Check sheet for the modelled part. Datum: model origin and axes. Units: mm. Face numbers are marked on the shaded views. A direction names the side the tool comes from. Round coordinates to 2 decimals unless told otherwise and drop trailing zeros. Order: outer loops, then holes, each group sorted by start corner. A loop starts at its lowest first (then second) coordinate and runs counter-clockwise, first axis right, second up. Notation, with made-up numbers: (-17.75, -11) -> (-4.75, -11) arc R27 cw to (-4.75, 18) -> close; hole circle Ø4 at (49, 19.5). An arc over 180 degrees is marked (long way). Answer in a Markdown table with one row per item.
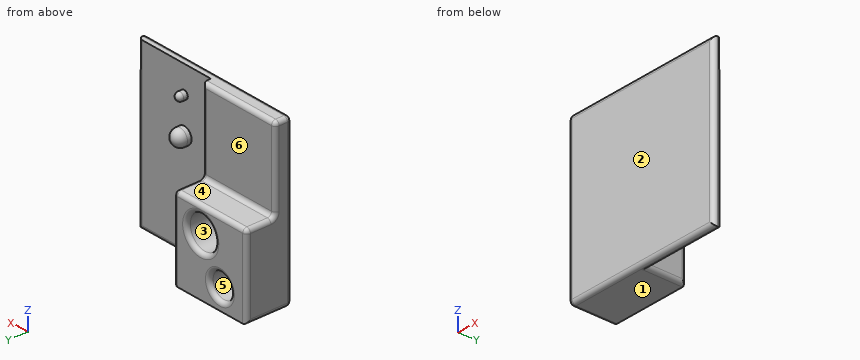
from build123d import *

# Parameters (mm, degrees)
SKETCH1_W           = 10
SKETCH1_H           = 20
BOSS_EXTRUDE1_DEPTH = 2
SKETCH2_W           = 10
SKETCH2_H           = 20
BOSS_EXTRUDE2_DEPTH = 1
SKETCH3_R           = 0.5
BOSS_EXTRUDE3_DEPTH = 1
FILLET1_R           = 0.5
SKETCH4_R           = 1
BOSS_EXTRUDE4_DEPTH = 1.5
FILLET2_R           = 1
SKETCH5_W           = 10
SKETCH5_H           = 10
BOSS_EXTRUDE5_DEPTH = 3.5
SKETCH7_R           = 1.5
CUT_EXTRUDE1_DEPTH  = 4
SKETCH8_R           = 2
CUT_EXTRUDE2_DEPTH  = 5
FILLET3_R           = 0.5


with BuildPart() as part:
    # Sketch1 → Boss-Extrude1 (new body)
    with BuildSketch(Plane(origin=(0, 0, 0), x_dir=(1, 0, 0), z_dir=(0, 1, 0))):
        with Locations((5, 10)):
            Rectangle(SKETCH1_W, SKETCH1_H)
    extrude(amount=BOSS_EXTRUDE1_DEPTH)

    # Sketch2 → Boss-Extrude2 (add)
    with BuildSketch(Plane(origin=(0, 0, 0), x_dir=(1, 0, 0), z_dir=(0, 1, 0))):
        with Locations((15, 10)):
            Rectangle(SKETCH2_W, SKETCH2_H)
    extrude(amount=BOSS_EXTRUDE2_DEPTH)

    # Sketch3 → Boss-Extrude3 (add)
    with BuildSketch(Plane(origin=(0, 1, 0), x_dir=(1, 0, 0), z_dir=(0, 1, 0))):
        with Locations(Location((13.691502903, 3.252748725, 0), (0, 0, 90))):
            Circle(SKETCH3_R)
    extrude(amount=BOSS_EXTRUDE3_DEPTH)

    # Fillet1
    fillet1_edges = [part.edges().sort_by_distance(p)[0] for p in [
        (13.691502903, 2, -2.752748725),
    ]]
    fillet(fillet1_edges, radius=FILLET1_R)

    # Sketch4 → Boss-Extrude4 (add)
    with BuildSketch(Plane(origin=(0, 1, 0), x_dir=(1, 0, 0), z_dir=(0, 1, 0))):
        with Locations(Location((13.672959069, 7.53387034, 0), (0, 0, 90))):
            Circle(SKETCH4_R)
    extrude(amount=BOSS_EXTRUDE4_DEPTH)

    # Fillet2
    fillet2_edges = [part.edges().sort_by_distance(p)[0] for p in [
        (13.672959069, 2.5, -6.53387034),
    ]]
    fillet(fillet2_edges, radius=FILLET2_R)

    # Sketch5 → Boss-Extrude5 (add)
    with BuildSketch(Plane(origin=(0, 2, 0), x_dir=(1, 0, 0), z_dir=(0, 1, 0))):
        with Locations((5, 15)):
            Rectangle(SKETCH5_W, SKETCH5_H)
    extrude(amount=BOSS_EXTRUDE5_DEPTH)

    # Sketch7 → Cut-Extrude1 (cut)
    with BuildSketch(Plane(origin=(0, 5.5, 0), x_dir=(1, 0, 0), z_dir=(0, 1, 0))):
        with Locations(Location((3.651027896, 17.503330669, 0), (0, 0, 270))):
            Circle(SKETCH7_R)
    extrude(amount=-CUT_EXTRUDE1_DEPTH, mode=Mode.SUBTRACT)

    # Sketch8 → Cut-Extrude2 (cut)
    with BuildSketch(Plane(origin=(0, 5.5, 0), x_dir=(1, 0, 0), z_dir=(0, 1, 0))):
        with Locations(Location((6.300805509, 13.043308943, 0), (0, 0, 270))):
            Circle(SKETCH8_R)
    extrude(amount=-CUT_EXTRUDE2_DEPTH, mode=Mode.SUBTRACT)

    # Fillet3
    fillet3_edges = [part.edges().sort_by_distance(p)[0] for p in [
        (0, 2, -5),
        (20, 0, -10),
        (20, 1, -10),
        (10, 0, -20),
        (0, 0, -10),
        (10, 0, 0),
        (0, 1, 0),
        (5, 2, 0),
        (5, 2, -10),
        (10, 2, -5),
        (15, 1, -20),
        (0, 2.75, -20),
        (10, 3.25, -20),
        (10, 5.5, -15),
        (10, 3.75, -10),
        (0, 3.75, -10),
        (0, 5.5, -15),
        (5, 5.5, -10),
        (6.300805509, 5.5, -15.043308943),
        (3.651027896, 5.5, -19.003330669),
    ]]
    fillet(fillet3_edges, radius=FILLET3_R - 0.0001)  # a hair under: the kernel refuses the full size


solid = part.part
Item 1: Cross-section at B-B (y = 4.3). Record the boundary of the cut face in (x, z), and give its area (3 significant figures).
Result sheet:
| item | result |
|---|---|
| outline | (0, -19.5) arc R0.5 ccw to (0.5, -20) -> (9.5, -20) arc R0.5 ccw to (10, -19.5) -> (10, -10.5) arc R0.5 ccw to (9.5, -10) -> (0.5, -10) arc R0.5 ccw to (0, -10.5) -> close; hole circle Ø3 at (3.65, -17.5); hole circle Ø4 at (6.3, -13.04) |
| area | 80.2 mm^2 |
Item 2: Depth check by flat-ended pin: P1, Ø5, axis at x = 6.3, z = -13.04, coming from the +Y side; P2, Ø7.5, axis at x = 14, z = -11, coming from the +Y side; P3, Ø1.5, axis at x = 16.5, z = -2, coming from the +Y side; P4, Ø4, axis at x = 6, z = -5.5, coming from the +Y side. Enter the tip coordinate at first touch or a pass-through.
Result sheet:
| item | result |
|---|---|
| P1 | stops at y = 5.5 |
| P2 | stops at y = 2.5 |
| P3 | stops at y = 1 |
| P4 | stops at y = 2 |
Item 3: Set-up check for the marked faces 4, 5 and 6: record each of +Z, -Z, +X, -X, +Y, -Y from which the full face is reachable in a straight line by a thin tool's end or side.
Result sheet:
| item | result |
|---|---|
| face 4 | +Z, +X, -X, +Y |
| face 5 | +Y |
| face 6 | +Z, -X, +Y |
Item 4: Scan lines: line 1 (Z direction, x = 3.75, y = 3.65); line 2 (Y direction, x = 14.75, z = -18); line 3 (Y direction, x = 9, z = -6.5). Record each from-to range of solid material in increasing order. Write a range as [from, to].
Result sheet:
| item | result |
|---|---|
| line 1 | z = [-20, -19], [-16.01, -10] |
| line 2 | y = [0, 1] |
| line 3 | y = [0, 2] |
Item 5: Mould release check, pull along Z, two halves, no side actions. Record for the marked faces 1, 2 and 3: pulls with the +Z half, pulls with the -Z half, needs draft (parallel to the pull), parting line crosses it, or undercut.
Result sheet:
| item | result |
|---|---|
| face 1 | pulls with the -Z half |
| face 2 | needs draft |
| face 3 | undercut |
